Part model, mm, in its own coordinate system. A direction names the side the tool comes from. Give positions to 0.01 mm unless a question says otherwise; leave off trailing zeros. Write each loop counter-clockwise with the first axis right and the second up, starting at its lowest first coordinate (ties: lowest second). Pieces come first, ordered by that corner, then holes. Notation, with made-up numbers: M 79.5,-18 L 137.5,-18 A22 ccw 137.5,-5 Z; hole C 32,73 d11. An arc over 180 degrees is marked long. Use a Markdown table: item, result.
```python
from build123d import *

# Parameters (mm, degrees)
F0_W     = 101.6
F0_H     = 50.8
F1_DEPTH = 6.35
F3_DEPTH = 0.381
F5_DEPTH = 5.969
F6_R     = 2.032
F7_DEPTH = 6.35


with BuildPart() as f1:
    # F0 (on Top) → F1 (new body)
    with BuildSketch(Plane.XY):
        with Locations((50.8, 25.4)):
            Rectangle(F0_W, F0_H)
    extrude(amount=F1_DEPTH)

    # F2 (on face) → F3 (cut)
    with BuildSketch(Plane.XY.offset(6.35)):
        with BuildLine():
            ThreePointArc((12.446, 15.621), (14.6910640303, 14.6910640303), (15.621, 12.446))
            Line((15.621, 12.446), (85.979, 12.446))
            ThreePointArc((85.979, 12.446), (86.9089359697, 14.6910640303), (89.154, 15.621))
            Line((89.154, 15.621), (89.154, 35.179))
            ThreePointArc((89.154, 35.179), (86.9089359697, 36.1089359697), (85.979, 38.354))
            Line((85.979, 38.354), (15.621, 38.354))
            ThreePointArc((15.621, 38.354), (14.6910640303, 36.1089359697), (12.446, 35.179))
            Line((12.446, 35.179), (12.446, 15.621))
        make_face()
        with BuildLine():
            Line((89.154, 38.354), (89.154, 35.179))
            ThreePointArc((89.154, 35.179), (91.3990640303, 36.1089359697), (92.329, 38.354))
            ThreePointArc((92.329, 38.354), (89.154, 41.529), (85.979, 38.354))
            Line((85.979, 38.354), (89.154, 38.354))
        make_face()
        with BuildLine():
            ThreePointArc((85.979, 38.354), (86.9089359697, 36.1089359697), (89.154, 35.179))
            Line((89.154, 35.179), (89.154, 38.354))
            Line((89.154, 38.354), (85.979, 38.354))
        make_face()
        with BuildLine():
            Line((12.446, 38.354), (12.446, 35.179))
            ThreePointArc((12.446, 35.179), (14.6910640303, 36.1089359697), (15.621, 38.354))
            Line((15.621, 38.354), (12.446, 38.354))
        make_face()
        with BuildLine():
            ThreePointArc((15.621, 38.354), (10.2009359697, 40.5990640303), (12.446, 35.179))
            Line((12.446, 35.179), (12.446, 38.354))
            Line((12.446, 38.354), (15.621, 38.354))
        make_face()
        with BuildLine():
            Line((89.154, 12.446), (85.979, 12.446))
            ThreePointArc((85.979, 12.446), (89.154, 9.271), (92.329, 12.446))
            ThreePointArc((92.329, 12.446), (91.3990640303, 14.6910640303), (89.154, 15.621))
            Line((89.154, 15.621), (89.154, 12.446))
        make_face()
        with BuildLine():
            ThreePointArc((89.154, 15.621), (86.9089359697, 14.6910640303), (85.979, 12.446))
            Line((85.979, 12.446), (89.154, 12.446))
            Line((89.154, 12.446), (89.154, 15.621))
        make_face()
        with BuildLine():
            Line((15.621, 12.446), (12.446, 12.446))
            Line((12.446, 12.446), (12.446, 15.621))
            ThreePointArc((12.446, 15.621), (10.2009359697, 10.2009359697), (15.621, 12.446))
        make_face()
        with BuildLine():
            Line((12.446, 15.621), (12.446, 12.446))
            Line((12.446, 12.446), (15.621, 12.446))
            ThreePointArc((15.621, 12.446), (14.6910640303, 14.6910640303), (12.446, 15.621))
        make_face()
    extrude(amount=-F3_DEPTH, mode=Mode.SUBTRACT)

    # F4 (on face) → F5 (cut, through all)
    with BuildSketch(Plane.XY.offset(5.969)):
        with BuildLine():
            ThreePointArc((14.986, 17.526), (15.7299487758, 15.7299487758), (17.526, 14.986))
            Line((17.526, 14.986), (83.566, 14.986))
            ThreePointArc((83.566, 14.986), (85.3620512242, 15.7299487758), (86.106, 17.526))
            Line((86.106, 17.526), (86.106, 32.766))
            ThreePointArc((86.106, 32.766), (85.3620512242, 34.5620512242), (83.566, 35.306))
            Line((83.566, 35.306), (17.526, 35.306))
            ThreePointArc((17.526, 35.306), (15.7299487758, 34.5620512242), (14.986, 32.766))
            Line((14.986, 32.766), (14.986, 17.526))
        make_face()
    extrude(amount=-F5_DEPTH, mode=Mode.SUBTRACT)

    # F6 (on face) → F7 (cut, through all)
    with BuildSketch(Plane.XY.offset(6.35)):
        with Locations((6.35, 44.45)):
            Circle(F6_R)
        with Locations((50.8, 44.45)):
            Circle(F6_R)
        with Locations((95.25, 44.45)):
            Circle(F6_R)
        with Locations((95.25, 6.35)):
            Circle(F6_R)
        with Locations((50.8, 6.35)):
            Circle(F6_R)
        with Locations((6.35, 6.35)):
            Circle(F6_R)
    extrude(amount=-F7_DEPTH, mode=Mode.SUBTRACT)


solid = f1.part
```
1. Cut at A-A, the plane x = 81. Give the cut face in (y, z), then the cut area to 3 significant figures.
Findings below:
| item | result |
|---|---|
| outline | M 0,0 L 14.99,0 L 14.99,5.97 L 12.45,5.97 L 12.45,6.35 L 0,6.35 Z; M 35.31,0 L 50.8,0 L 50.8,6.35 L 38.35,6.35 L 38.35,5.97 L 35.31,5.97 Z |
| area | 191 mm2 |
2. Cut at B-B, the plane y = 6.35. Give the cut face in (x, z).
Findings below:
| item | result |
|---|---|
| outline | M 0,0 L 4.32,0 L 4.32,6.35 L 0,6.35 Z; M 8.38,0 L 48.77,0 L 48.77,6.35 L 8.38,6.35 Z; M 52.83,0 L 93.22,0 L 93.22,6.35 L 52.83,6.35 Z; M 97.28,0 L 101.6,0 L 101.6,6.35 L 97.28,6.35 Z |
3. Cut at D-D, the plane z = 4.75. Give the cut face in (x, y), then the cut area to 3 significant figures.
Findings below:
| item | result |
|---|---|
| outline | M 0,0 L 101.6,0 L 101.6,50.8 L 0,50.8 Z; hole C 6.35,6.35 d4.06; hole C 6.35,44.45 d4.06; hole M 14.99,17.53 A2.54 ccw 17.53,14.99 L 83.57,14.99 A2.54 ccw 86.11,17.53 L 86.11,32.77 A2.54 ccw 83.57,35.31 L 17.53,35.31 A2.54 ccw 14.99,32.77 Z; hole C 50.8,6.35 d4.06; hole C 50.8,44.45 d4.06; hole C 95.25,6.35 d4.06; hole C 95.25,44.45 d4.06 |
| area | 3,640 mm2 |
4. Drill centre lines: L1, parallel to Y at x = 95.25, z = 3.5; L2, parallel to Y at x = 54, z = 2.25; L3, parallel to Y at x = 50.8, z = 4. Where is each one in solid material? Low to high.
Findings below:
| item | result |
|---|---|
| L1 | 0 to 4.32, 8.38 to 42.42, 46.48 to 50.8 |
| L2 | 0 to 14.99, 35.31 to 50.8 |
| L3 | 0 to 4.32, 8.38 to 14.99, 35.31 to 42.42, 46.48 to 50.8 |
5. Tool access for faces 1 (the cylindrical face through (85.382, 34.542, 3.026)), 2 (the flat face through (50, 9, 6.35)): list every direction of +Z, -Z, +X, -X, +Y, -Y with a clear straight run to the whole face (end or side of a thin tool).
Findings below:
| item | result |
|---|---|
| face 1 | +Z, -Z |
| face 2 | +Z, +X, -X, +Y, -Y |
6. Drop flat-ended pins along their axis: P1, Ø10, axis at x = 12.446, y = 12.446, coming from the +Z side; P2, Ø1.5, axis at x = 13, y = 10.5, coming from the +Z side. Give the stop position or say it passes through.
Findings below:
| item | result |
|---|---|
| P1 | z = 6.35 |
| P2 | z = 5.97 |
7. Two-plate mould, pull along Y, no slides. Class faces 3 (the cylindrical face through (15.71, 15.75, 3.03)), 4 (the flat face through (50, 14, 0)), 5 (the flat face through (50, 50.8, 3)), 6 (the cylindrical face through (10.128, 10.276, 6.162)): released by +Y, released by -Y, zero draft, split by the parting line, or undercut.
Findings below:
| item | result |
|---|---|
| face 3 | undercut |
| face 4 | zero draft |
| face 5 | released by +Y |
| face 6 | undercut |
8. Cut at C-C, the plane x = 95.25. Give the cut face in (y, z), then the cut area to 3 significant figures.
Findings below:
| item | result |
|---|---|
| outline | M 0,0 L 4.32,0 L 4.32,6.35 L 0,6.35 Z; M 8.38,0 L 42.42,0 L 42.42,6.35 L 8.38,6.35 Z; M 46.48,0 L 50.8,0 L 50.8,6.35 L 46.48,6.35 Z |
| area | 271 mm2 |
